For this review, take the finished solid that the model builds, in its own axes (mm). A direction names the side the tool comes from. Coordinates: 2 decimals unless noted, no trailing zeros. Loops run counter-clockwise (first coordinate to the right, second up) from the corner with the lowest first, then second, coordinate; pieces in that order, holes last. Notation, with made-up numbers: M -24,6 L -13,6 A14 ccw -13,11 Z; hole C 30,4.5 d8. An arc over 180 degrees is marked long. Answer as a JSON object with one key per item and string values. Group by question number.
Item 1: Add section D-D (x = 141). State the section outline as (y, z) points.
Item 2: Add section C-C (y = 80.5). State the section outline as (x, z) points, then the cut area to 3 significant figures.
Item 3: Tool access review of faces 1 (the face through (140, 101.6, 13)), 2 (the face through (203.2, 25, 13)), 3 (the face through (64, 101.6, 13)), 4 (the face through (101.321, 114.297, 12.522)), 5 (the face through (102.159, 126.994, 12.522)): name each direction out of +Z, -Z, +X, -X, +Y, -Y from which nothing blocks a thin tool from reaching the whole face with its end or side.
Item 4: Add section A-A (z = 15.25). State the section outline as (x, y) points.
Item 5: Wall thickness on L1, parallel to Y at x = 56, z = 4.25; L2, parallel to X at y = 110, z = 2.25; L3, parallel to Y at x = 92, z = 12: over which ranges is each line inside the solid? List them lowest first. Write a range as from..to.
Item 6: Add section B-B (x = 101.6). State the section outline as (y, z) points.
Item 7: Mouldability with a two-part tool opening along Y and no side actions: class faces 6 (the face through (100, 0, 13)), 7 (the face through (102, 101.6, 13)), 8 (the face through (100, 50, 25.4)) as +Y half, -Y half, draft (parallel to the pull), parting line (faces both ways), or undercut.
Item 8: Insertion check: pin 1 (6 mm diameter, centred on x = 48, z = 10.5, fed in from +Y); pin 2 (12 mm diameter, centred on y = 25.5, z = 8, fed in from -X); pin 3 (3 mm diameter, centred on x = 105.5, z = 4.5, fed in from +Y); pin 4 (6 mm diameter, centred on y = 83, z = 18, fed in from +X). Each pin has a flat end and moves straight along its axis. Give the tip position at first contact, or say it passes through.
from build123d import *

# Parameters (mm, degrees)
F1_DEPTH = 25.4


with BuildPart() as f1:
    # F0 (on Top) → F1 (new body)
    with BuildSketch(Plane.XY):
        with BuildLine():
            Line((0, 50.8), (0, 0))
            Line((0, 0), (203.2, 0))
            Line((203.2, 0), (203.2, 50.8))
            Line((203.2, 50.8), (152.4, 101.6))
            Line((152.4, 101.6), (127, 101.6))
            ThreePointArc((127, 101.6), (101.6, 127), (76.2, 101.6))
            Line((76.2, 101.6), (50.8, 101.6))
            Line((50.8, 101.6), (0, 50.8))
        make_face()
        with BuildLine():
            ThreePointArc((88.9, 101.6), (101.6, 114.3), (114.3, 101.6))
            Line((114.3, 101.6), (88.9, 101.6))
        make_face(mode=Mode.SUBTRACT)
    extrude(amount=F1_DEPTH)


solid = f1.part
From the geometry:
{
 "1": {"outline": "M 0,0 L 101.6,0 L 101.6,25.4 L 0,25.4 Z"},
 "2": {"outline": "M 29.7,0 L 173.5,0 L 173.5,25.4 L 29.7,25.4 Z", "area": "3,650 mm²"},
 "3": {"face 1": "+Z, -Z, +X, +Y", "face 2": "+Z, -Z, +X, +Y, -Y", "face 3": "+Z, -Z, -X, +Y", "face 4": "+Z, -Z", "face 5": "+Z, -Z, +Y"},
 "4": {"outline": "M 0,0 L 203.2,0 L 203.2,50.8 L 152.4,101.6 L 127,101.6 A25.4 ccw 76.2,101.6 L 50.8,101.6 L 0,50.8 Z; hole M 88.9,101.6 L 114.3,101.6 A12.7 ccw Z"},
 "5": {"L1": "y = 0..101.6", "L2": "x = 77.63..92.07, 111.13..125.57", "L3": "y = 0..101.6, 109.91..125.12"},
 "6": {"outline": "M 0,0 L 101.6,0 L 101.6,25.4 L 0,25.4 Z; M 114.3,0 L 127,0 L 127,25.4 L 114.3,25.4 Z"},
 "7": {"face 6": "-Y half", "face 7": "undercut", "face 8": "draft"},
 "8": {"pin 1": "stops at y = 101.6", "pin 2": "stops at x = 0", "pin 3": "stops at y = 126.89", "pin 4": "stops at x = 174"}
}
